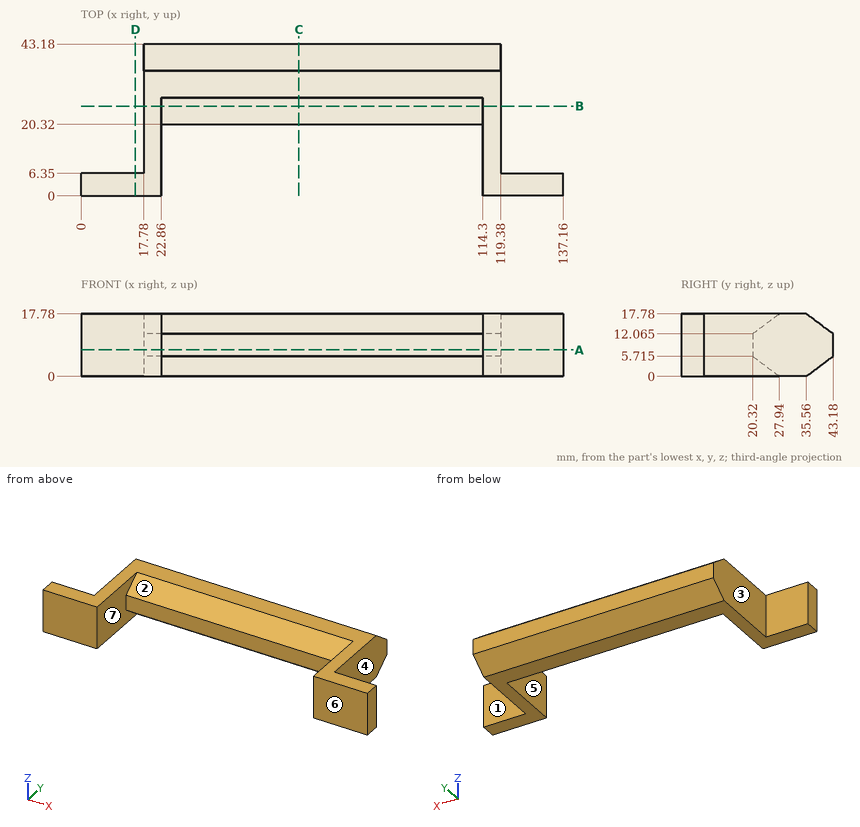
Source: three-view drawing plus pictorial views. Frame: mm from the lowest corner of the part. A direction names the side the tool comes from. Give positions to 0.01 mm unless a question says otherwise; leave off trailing zeros. Order: outer loops, then holes, each group sorted by start corner. A loop starts at its lowest first (then second) coordinate and runs counter-clockwise, first axis right, second up. Notation, with made-up numbers: M -30,53 L -9,53 A36 ccw -9,88 Z; hole C 36,41 d3. An arc over 180 degrees is marked long. Return JSON: item names as keys, results as strings.
Item 1: Cut plane B-B (y = 25.5). Return loops of the section in (x, z).
Solutions:
{"outline": "M 17.78,0 L 22.86,0 L 22.86,1.83 L 114.3,1.83 L 114.3,0 L 119.38,0 L 119.38,17.78 L 114.3,17.78 L 114.3,15.95 L 22.86,15.95 L 22.86,17.78 L 17.78,17.78 Z"}
Item 2: Ray query, probe 1 along X at (y, z) = (13, 1.75); probe 2 along X at (y, z) = (3, 7.25); probe 3 along Y at (x, z) = (25, 8.75). Return the intervals inside material, ascending.
Solutions:
{"probe 1": "17.78 to 22.86, 114.3 to 119.38", "probe 2": "0 to 22.86, 114.3 to 137.16", "probe 3": "20.32 to 43.18"}
Item 3: First-contact query: P1, Ø1, axis at y = 24.5, z = 4, coming from the -X side; P2, Ø4, axis at y = 34.5, z = 7, coming from the +X side; P3, Ø1, axis at x = 50.5, z = 11.5, coming from the -Y side. Flat tips, straight axial feed; report the tip coordinate or a pass-through.
Solutions:
{"P1": "x = 17.78", "P2": "x = 119.38", "P3": "y = 20.32"}
Item 4: Access query for the marked faces 1, 2 and 3. Directions: +Z, -Z, +X, -X, +Y, -Y. A direction counts if a zero-diameter tool reaches every point of the face in a straight line with its end or side. Return the directions, or none.
Solutions:
{"face 1": "+Z, -Z, +X, +Y", "face 2": "+Z, -Y", "face 3": "+Z, -Z, -X, +Y"}
Item 5: Cut plane D-D (x = 15.5). Return loops of the section in (y, z).
Solutions:
{"outline": "M 0,0 L 6.35,0 L 6.35,17.78 L 0,17.78 Z"}
Item 6: Pull-direction query (X, two-part tool) for the marked faces 4, 5, 6 and 7; classes: +X half, -X half, draft (parallel to the pull), parting line (faces both ways), or undercut.
Solutions:
{"face 4": "+X half", "face 5": "undercut", "face 6": "draft", "face 7": "undercut"}
Item 7: Cut plane C-C (x = 62). Return loops of the section in (y, z) (3 decimals), then the cut area to 3 significant figures.
Solutions:
{"outline": "M 20.32,5.715 L 27.94,0 L 35.56,0 L 43.18,5.715 L 43.18,12.065 L 35.56,17.78 L 27.94,17.78 L 20.32,12.065 Z", "area": "319 mm^2"}
Item 8: Cut plane A-A (z = 7.5). Return loops of the section in (x, y), then the cut area to 3 significant figures.
Solutions:
{"outline": "M 0,0 L 22.86,0 L 22.86,20.32 L 114.3,20.32 L 114.3,0 L 137.16,0 L 137.16,6.35 L 119.38,6.35 L 119.38,43.18 L 17.78,43.18 L 17.78,6.35 L 0,6.35 Z", "area": "2,750 mm^2"}
